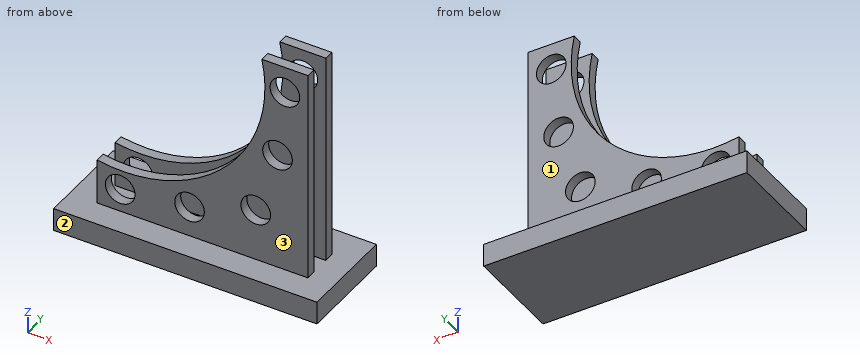
```python
from build123d import *

# Parameters (mm, degrees)
F0_W     = 320
F0_H     = 60
F1_DEPTH = 360
F2_R     = 22.5
F3_DEPTH = 60
F5_DEPTH = 101.068698
F6_W     = 30
F6_H     = 360
F7_DEPTH = 320
F8_W     = 399.738486
F8_H     = 149.227709
F9_DEPTH = 35


with BuildPart() as f1:
    # F0 (on Top) → F1 (new body)
    with BuildSketch(Plane.XY):
        with Locations((-160, -71.068698)):
            Rectangle(F0_W, F0_H)
    extrude(amount=F1_DEPTH)

    # F2 (on face) → F3 (cut, through all)
    with BuildSketch(Plane.XZ.offset(101.068698)):
        with Locations((-35, 320)):
            Circle(F2_R)
        with Locations((-285, 70)):
            Circle(F2_R)
        with Locations((-179.76, 81.2)):
            Circle(F2_R)
        with Locations((-79.24, 114.3)):
            Circle(F2_R)
        with Locations((-46.2, 214.76)):
            Circle(F2_R)
    extrude(amount=-F3_DEPTH, mode=Mode.SUBTRACT)

    # F4 (on Front) → F5 (cut, through all)
    with BuildSketch(Plane.XZ):
        with BuildLine():
            Line((-320, 360), (-320, 104.046823))
            ThreePointArc((-320, 104.046823), (-126.506917, 165.123399), (-70, 360))
            Line((-70, 360), (-320, 360))
        make_face()
    extrude(amount=F5_DEPTH, mode=Mode.SUBTRACT)

    # F6 (on Right) → F7 (cut, through all)
    with BuildSketch(Plane.YZ):
        with Locations((-71.068698, 180)):
            Rectangle(F6_W, F6_H)
    extrude(amount=-F7_DEPTH, mode=Mode.SUBTRACT)

    # F8 (on face) → F9 (join)
    with BuildSketch(Plane(origin=(0, 0, 0), x_dir=(1, 0, 0), z_dir=(0, 0, -1))):
        with Locations((-162.054332, 66.393896)):
            Rectangle(F8_W, F8_H)
    extrude(amount=-F9_DEPTH)


solid = f1.part
```
Design review of the part built by this model. Coordinates are the model's own, in mm. Face numbers are marked on the shaded views. A direction names the side the tool comes from. Give positions to 0.01 mm unless a question says otherwise; leave off trailing zeros. Order: outer loops, then holes, each group sorted by start corner. A loop starts at its lowest first (then second) coordinate and runs counter-clockwise, first axis right, second up. Notation, with made-up numbers: (24, 74) - (76, 74) arc R18 cw to (76, 81) - close; hole circle Ø10 at (62, 8.5). An arc over 180 degrees is marked (long way). Use a Markdown table: item, result. Add a question column.
(1) Machinability: for the marked faces 1, 2 and 3, which of the approach directions +Z, -Z, +X, -X, +Y, -Y give a long, thin tool a straight path to every point of the face, cutting with its end or side? Answer none if there is none.
(2) Clearance check with flat-ended pins moving along their axes: P1, Ø2, axis at x = -273.5, y = -26, coming from the +Z side; P2, Ø8, axis at x = -24.5, z = 269, coming from the +Y side; P3, Ø4.5, axis at y = -52, z = 54, coming from the -X side. State where each tip first meets the part, or that it passes through.
(3) Add section D-D on y = -119. Give the boundary of the cut face in (x, z).
(4) Add section A-A on z = 285.5. Give the boundary of the cut face in (x, y).
(5) Wall thickness on probe 1 along X at (y, z) = (-96.5, 68.5); probe 2 along Y at (x, z) = (-282.5, 99); probe 3 along Z at (x, y) = (-285, -91): over which ranges is each line inside the solid? List them lowest first. Write a range as [from, to].
(6) Add section B-B on x = -193. Give the boundary of the cut face in (y, z).
(7) Add section C-C on z = 114.3. Give the boundary of the cut face in (x, y), then the cut area to 3 significant figures.
Report:
| question | item | result |
|---|---|---|
| 1 | face 1 | +Z, +X, -X, +Y |
| 1 | face 2 | +Z, -Z, +X, -X, -Y |
| 1 | face 3 | +Z, +X, -X, -Y |
| 2 | P1 | stops at z = 35 |
| 2 | P2 | stops at y = -41.07 |
| 2 | P3 | stops at x = -320 |
| 3 | outline | (-361.92, 0) - (37.81, 0) - (37.81, 35) - (-361.92, 35) - close |
| 4 | outline | (-67.4, -101.07) - (0, -101.07) - (0, -86.07) - (-67.4, -86.07) - close; (-67.4, -56.07) - (0, -56.07) - (0, -41.07) - (-67.4, -41.07) - close |
| 5 | probe 1 | x = [-320, -307.45], [-262.55, -198.33], [-161.19, 0] |
| 5 | probe 2 | y = [-101.07, -86.07], [-56.07, -41.07] |
| 5 | probe 3 | z = [0, 47.5], [92.5, 100.4] |
| 6 | outline | (-141.01, 0) - (8.22, 0) - (8.22, 35) - (-41.07, 35) - (-41.07, 63.01) - (-56.07, 63.01) - (-56.07, 35) - (-86.07, 35) - (-86.07, 63.01) - (-101.07, 63.01) - (-101.07, 35) - (-141.01, 35) - close; (-101.07, 99.39) - (-86.07, 99.39) - (-86.07, 118.88) - (-101.07, 118.88) - close; (-56.07, 99.39) - (-41.07, 99.39) - (-41.07, 118.88) - (-56.07, 118.88) - close |
| 7 | outline | (-204.14, -101.07) - (-101.74, -101.07) - (-101.74, -86.07) - (-204.14, -86.07) - close; (-204.14, -56.07) - (-101.74, -56.07) - (-101.74, -41.07) - (-204.14, -41.07) - close; (-56.74, -101.07) - (0, -101.07) - (0, -86.07) - (-56.74, -86.07) - close; (-56.74, -56.07) - (0, -56.07) - (0, -41.07) - (-56.74, -41.07) - close |
| 7 | area | 4,770 mm² |
